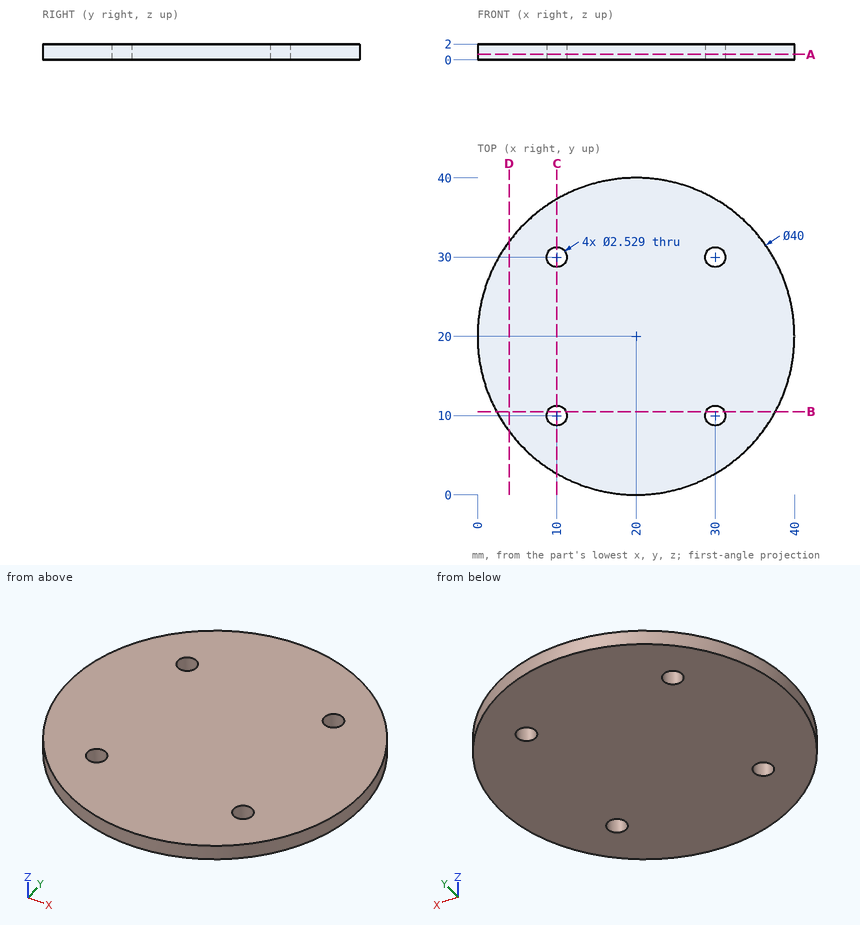
Input: dimensioned drawing with shaded views. Units: mm. Origin: part minimum x, y, z. Round coordinates to 2 decimals unless told otherwise and drop trailing zeros. Order: outer loops, then holes, each group sorted by start corner. A loop starts at its lowest first (then second) coordinate and runs counter-clockwise, first axis right, second up.
1. Cut plane A-A, the plane z = 0.7. Output: boundary loops of the cut face in (x, y), then the cut area to 3 significant figures.
The answers:
outline: circle Ø40 at (20, 20); hole circle Ø2.53 at (10, 10); hole circle Ø2.53 at (10, 30); hole circle Ø2.53 at (30, 10); hole circle Ø2.53 at (30, 30)
area: 1,240 mm2
2. Cut plane C-C, the plane x = 10. Output: boundary loops of the cut face in (y, z), then the cut area to 3 significant figures.
The answers:
outline: (2.68, 0) - (8.74, 0) - (8.74, 2) - (2.68, 2) - close; (11.26, 0) - (28.74, 0) - (28.74, 2) - (11.26, 2) - close; (31.26, 0) - (37.32, 0) - (37.32, 2) - (31.26, 2) - close
area: 59.2 mm2
3. Material intervals for line 1 (Y direction, x = 10, z = 1.8); line 2 (Y direction, x = 31, z = 1.05), sorted ascending.
The answers:
line 1: y = 2.68 to 8.74, 11.26 to 28.74, 31.26 to 37.32
line 2: y = 3.3 to 9.23, 10.77 to 29.23, 30.77 to 36.7
4. Cut plane D-D, the plane x = 4. Output: boundary loops of the cut face in (y, z), then the cut area to 3 significant figures.
The answers:
outline: (8, 0) - (32, 0) - (32, 2) - (8, 2) - close
area: 48.0 mm2
5. Cut plane B-B, the plane y = 10.5. Output: boundary loops of the cut face in (x, z).
The answers:
outline: (2.4, 0) - (8.84, 0) - (8.84, 2) - (2.4, 2) - close; (11.16, 0) - (28.84, 0) - (28.84, 2) - (11.16, 2) - close; (31.16, 0) - (37.6, 0) - (37.6, 2) - (31.16, 2) - close
